Build history of the part. All positions in model axes, mm. A direction names the side the tool comes from. Coordinates: 2 decimals unless noted, no trailing zeros. Loops run counter-clockwise (first coordinate to the right, second up) from the corner with the lowest first, then second, coordinate; pieces in that order, holes last. Notation, with made-up numbers: (-34.5, -22.5) - (19.5, -22.5) arc R25 cw to (19.5, 8.5) - close; hole circle Ø7 at (-10, -3.75). An arc over 180 degrees is marked (long way). One line per item, written item: value.
```python
from build123d import *

# Parameters (mm, degrees)
BOSS_EXTRUDE1_DEPTH = 5
SKETCH2_R           = 1.591812525
CUT_EXTRUDE1_DEPTH  = 37.400549446


with BuildPart() as part:
    # Sketch1 → Boss-Extrude1 (new body)
    with BuildSketch(Plane.XY):
        Polygon((-15, 15), (15, 15), (20, 15), (20, 2.5), (10, 2.5), (10, -2.5), (20, -2.5), (20, -15), (15, -15), (-15, -15), (-20, -15), (-20, -2.5), (-10, -2.5), (-10, 2.5), (-20, 2.5), (-20, 15), align=None)
    extrude(amount=BOSS_EXTRUDE1_DEPTH)

    # Sketch2 → Cut-Extrude1 (cut, through all)
    with BuildSketch(Plane(origin=(0, 15, 0), x_dir=(1, 0, 0), z_dir=(0, 1, 0))):
        with Locations(Location((-15, -2.5, 0), (0, 0, 180))):
            Circle(SKETCH2_R)
    cut_extrude1 = extrude(amount=-CUT_EXTRUDE1_DEPTH, mode=Mode.SUBTRACT)

    # Mirror1: Cut-Extrude1 across plane
    add(cut_extrude1.mirror(Plane(origin=(0, 0, 0), x_dir=(0, 0, 1), z_dir=(1, 0, 0))), mode=Mode.SUBTRACT)


solid = part.part
```
Item 1: Probe probe 1 along X at (y, z) = (8, 2.6); probe 2 along Y at (x, z) = (-11.5, 4.3); probe 3 along X at (y, z) = (8, 3.45). List the from-to ranges inside material, lowest first. Write a range as from..to.
Check result:
probe 1: x = -20..-16.59, -13.41..13.41, 16.59..20
probe 2: y = -15..-2.5, 2.5..15
probe 3: x = -20..-16.28, -13.72..13.72, 16.28..20
Item 2: Tool access for faces 1 (the face through (-14, 2.5, 1)), 2 (the face through (20, -9, 2)), 3 (the face through (14, -2.5, 1)): list every direction of +Z, -Z, +X, -X, +Y, -Y with a clear straight run to the whole face (end or side of a thin tool).
Check result:
face 1: +Z, -Z, -X
face 2: +Z, -Z, +X, +Y, -Y
face 3: +Z, -Z, +X
Item 3: Cut at C-C, the plane y = -6.25. Write the cut outline in (x, z), then the cut area to 3 significant figures.
Check result:
outline: (-20, 0) - (20, 0) - (20, 5) - (-20, 5) - close; hole circle Ø3.18 at (-15, 2.5); hole circle Ø3.18 at (15, 2.5)
area: 184 mm^2
Item 4: Cut at B-B, the plane z = 2.5. Write the cut outline in (x, y).
Check result:
outline: (-20, -15) - (-16.59, -15) - (-16.59, -2.5) - (-20, -2.5) - close; (-20, 2.5) - (-16.59, 2.5) - (-16.59, 15) - (-20, 15) - close; (-13.41, -15) - (13.41, -15) - (13.41, -2.5) - (10, -2.5) - (10, 2.5) - (13.41, 2.5) - (13.41, 15) - (-13.41, 15) - (-13.41, 2.5) - (-10, 2.5) - (-10, -2.5) - (-13.41, -2.5) - close; (16.59, -15) - (20, -15) - (20, -2.5) - (16.59, -2.5) - close; (16.59, 2.5) - (20, 2.5) - (20, 15) - (16.59, 15) - close
Item 5: Pull direction Y, two halves, no side cores. Call faces 4 (the face through (0, 0, 0)), 5 (the face through (0, -15, 2)), 6 (the face through (-16, -2.5, 1)): released by +Y, released by -Y, zero draft, split by the parting line, or undercut.
Check result:
face 4: zero draft
face 5: released by -Y
face 6: undercut
Item 6: Drop flat-ended pins along their axis: P1, Ø1.5, axis at x = -15.5, z = 3.5, coming from the -Y side; P2, Ø2.5, axis at y = 1, z = 2.5, coming from the -X side; P3, Ø1.5, axis at y = 0, z = 2, coming from the +X side. Give the stop position or say it passes through.
Check result:
P1: stops at y = -15
P2: stops at x = -10
P3: stops at x = 10
Item 7: Cut at A-A, the plane x = 15. Write the cut outline in (y, z), then the cut area to 3 significant figures.
Check result:
outline: (-15, 0) - (-2.5, 0) - (-2.5, 0.91) - (-15, 0.91) - close; (-15, 4.09) - (-2.5, 4.09) - (-2.5, 5) - (-15, 5) - close; (2.5, 0) - (15, 0) - (15, 0.91) - (2.5, 0.91) - close; (2.5, 4.09) - (15, 4.09) - (15, 5) - (2.5, 5) - close
area: 45.4 mm^2
